Design review of the part built by this model. Coordinates are the model's own, in mm. Round coordinates to 2 decimals unless told otherwise and drop trailing zeros. Write each loop counter-clockwise with the first axis right and the second up, starting at its lowest first coordinate (ties: lowest second). Pieces come first, ordered by that corner, then holes.
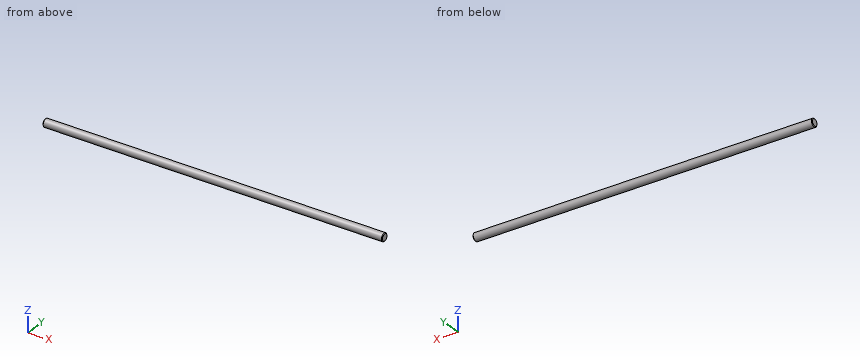
from build123d import *

# Parameters (mm, degrees)
SKETCH1_R           = 6.35
BOSS_EXTRUDE1_DEPTH = 268
CHAMFER1_SIZE       = 1
CHAMFER2_SIZE       = 1


with BuildPart() as part:
    # Sketch1 → Boss-Extrude1 (new body, symmetric)
    with BuildSketch(Plane(origin=(0, 0, 0), x_dir=(0, 0, -1), z_dir=(1, 0, 0))):
        Circle(SKETCH1_R)
    extrude(amount=BOSS_EXTRUDE1_DEPTH, both=True)

    # Chamfer1
    chamfer1_edges = [part.edges().sort_by_distance(p)[0] for p in [
        (-268, 0, 6.35),
    ]]
    chamfer(chamfer1_edges, length=CHAMFER1_SIZE)

    # Chamfer2
    chamfer2_edges = [part.edges().sort_by_distance(p)[0] for p in [
        (268, 0, 6.35),
    ]]
    chamfer(chamfer2_edges, length=CHAMFER2_SIZE)


solid = part.part
1) Add section A-A on x = 185.5. State the section outline as (y, z) points.
2) For P1, Ø5, axis at x = 177, z = -4, coming from the -Y side; P2, Ø6, axis at x = -139, z = 3.5, coming from the +Y side; P3, Ø1.5, axis at x = 149.5, y = -5, coming from the -Z side, all flat-tipped, find the tip position at first contact; note any pin that passes through.
3) For line 1 along Z through (x, y) = (234.5, 0.75); line 2 along Y through (x, z) = (207, -3.5); line 3 along Y through (x, z) = (71, -3.25), list the stretches that pass through material, from the lowest coordinate up.
Computed:
1. outline: circle Ø12.7 at (0, 0)
2. P1: stops at y = -6.17
2. P2: stops at y = 6.33
2. P3: stops at z = -4.72
3. line 1: z = -6.31 to 6.31
3. line 2: y = -5.3 to 5.3
3. line 3: y = -5.46 to 5.46
